Model file for the job. Use its own axes, mm. A direction names the side the tool comes from. Coordinates: 2 decimals unless noted, no trailing zeros. Order: outer loops, then holes, each group sorted by start corner. A loop starts at its lowest first (then second) coordinate and runs counter-clockwise, first axis right, second up. Notation, with made-up numbers: (-29.5, 4.5) -> (19.5, 4.5) arc R28 ccw to (19.5, 30.5) -> close; hole circle Ø8 at (2, 45). An arc over 180 degrees is marked (long way). Return JSON: item names as keys, results as strings. Group by question number.
1) Cut at C-C (y = -84.5). Write the cut outline in (x, z), and give its area (3 significant figures).
2) Pull direction Z, two halves, no side cores. Call faces 6 (the flat face through (9, -69, -6.5)), 7 (the flat face through (34, -77, 0)), 8 (the flat face through (-12.45, -87.22, -2.94)): +Z half, -Z half, draft (parallel to the pull), parting line (faces both ways), or undercut.
3) Cut at A-A (z = 0). Write the cut outline in (x, y).
4) Cut at B-B (x = -12). Write the cut outline in (y, z).
5) Cut at D-D (z = 5). Write the cut outline in (x, y), and give its area (3 significant figures).
6) Probe line 1 (Y direction, x = -6, z = 3); line 2 (X direction, y = -74.5, z = -2); line 3 (X direction, y = -88.5, z = 0). List the from-to ranges inside material, lowest first.
7) Flat gauge pins, fed straight in: pin 1 (4 mm diameter, centred on y = -81, z = 2.5, fed in from +X); pin 2 (3.5 mm diameter, centred on y = -86.5, z = -0.5, fed in from -X); pin 3 (4.5 mm diameter, centred on x = 34.5, z = 1.5, fed in from -Y); pin 4 (1 mm diameter, centred on x = 5, z = 4, fed in from -Y). Where does each tip first touch, or does it go through?
8) Which spindle directions (+Z, -Z, +X, -X, +Y, -Y) get a long thin tool onto all of the face, cutting with end or side? Do faces 1 (the flat face through (16, -62, 0)), 2 (the flat face through (-6.5, -87, 0)), 3 (the flat face through (-1, -82, 0)), 4 (the flat face through (-15, -50.15, 0)), 5 (the flat face through (34, -59, 0)). Say none if no direction does.
from build123d import *

# Parameters (mm, degrees)
BOSS_EXTRUDE1_START = -3
SKETCH1_W           = 13
SKETCH1_H           = 42.2
BOSS_EXTRUDE1_DEPTH = 2
BOSS_EXTRUDE2_START = -87.25
SKETCH2_R           = 6.5
BOSS_EXTRUDE2_DEPTH = 2.1
BOSS_EXTRUDE3_START = -87.25
SKETCH3_W           = 18.2
SKETCH3_H           = 13
BOSS_EXTRUDE3_DEPTH = 2.1
CUT_EXTRUDE1_START  = -87.25
SKETCH4_R           = 3.55
CUT_EXTRUDE1_DEPTH  = 2.1
CUT_EXTRUDE2_START  = -87.25
CUT_EXTRUDE2_DEPTH  = 2.1
BOSS_EXTRUDE4_START = -48.65
SKETCH6_R           = 6.5
BOSS_EXTRUDE4_DEPTH = 1.5
BOSS_EXTRUDE5_START = -48.65
SKETCH7_W           = 18.2
SKETCH7_H           = 13
BOSS_EXTRUDE5_DEPTH = 1.5
CUT_EXTRUDE3_START  = -48.65
SKETCH8_R           = 2.95
CUT_EXTRUDE3_DEPTH  = 1.5
BOSS_EXTRUDE6_START = 17
SKETCH9_W           = 13
SKETCH9_H           = 12
BOSS_EXTRUDE6_DEPTH = 19
BOSS_EXTRUDE7_START = 34
SKETCH10_W          = 13
SKETCH10_H          = 18
BOSS_EXTRUDE7_DEPTH = 2


with BuildPart() as part:
    # Sketch1 → Boss-Extrude1 (new, symmetric)
    with BuildSketch(Plane(origin=(0, 0, 0), x_dir=(0, 0, -1), z_dir=(1, 0, 0)).offset(BOSS_EXTRUDE1_START)):
        with Locations((0, -68.25)):
            Rectangle(SKETCH1_W, SKETCH1_H)
    extrude(amount=BOSS_EXTRUDE1_DEPTH, both=True)



with BuildPart() as body_2:
    # Sketch2 → Boss-Extrude2 (new, symmetric)
    with BuildSketch(Plane(origin=(0, 0, 0), x_dir=(1, 0, 0), z_dir=(0, 1, 0)).offset(BOSS_EXTRUDE2_START)):
        with Locations(Location((-19.2, 0, 0), (0, 0, 270))):
            Circle(SKETCH2_R)
    extrude(amount=BOSS_EXTRUDE2_DEPTH, both=True)


with BuildPart() as part_1:
    add(part.part)

    add(body_2.part)  # Boss-Extrude3 merges body 2
    # Sketch3 → Boss-Extrude3 (add, symmetric)
    with BuildSketch(Plane(origin=(0, 0, 0), x_dir=(1, 0, 0), z_dir=(0, 1, 0)).offset(BOSS_EXTRUDE3_START)):
        with Locations((-10.1, 0)):
            Rectangle(SKETCH3_W, SKETCH3_H)
    extrude(amount=BOSS_EXTRUDE3_DEPTH, both=True)

    # Sketch4 → Cut-Extrude1 (cut, symmetric)
    with BuildSketch(Plane(origin=(0, 0, 0), x_dir=(1, 0, 0), z_dir=(0, 1, 0)).offset(CUT_EXTRUDE1_START)):
        with Locations(Location((-19.2, 0, 0), (0, 0, 270))):
            Circle(SKETCH4_R)
    extrude(amount=CUT_EXTRUDE1_DEPTH, both=True, mode=Mode.SUBTRACT)

    # Sketch5 → Cut-Extrude2 (cut, symmetric)
    with BuildSketch(Plane(origin=(0, 0, 0), x_dir=(1, 0, 0), z_dir=(0, 1, 0)).offset(CUT_EXTRUDE2_START)):
        Polygon((-19.2, -3.55), (-6.5, -2.403281405), (-6.5, 2.403281405), (-19.2, 3.55), align=None)
    extrude(amount=CUT_EXTRUDE2_DEPTH, both=True, mode=Mode.SUBTRACT)



with BuildPart() as body_2_2:
    # Sketch6 → Boss-Extrude4 (new, symmetric)
    with BuildSketch(Plane(origin=(0, 0, 0), x_dir=(1, 0, 0), z_dir=(0, 1, 0)).offset(BOSS_EXTRUDE4_START)):
        with Locations(Location((-19.2, 0, 0), (0, 0, 270))):
            Circle(SKETCH6_R)
    extrude(amount=BOSS_EXTRUDE4_DEPTH, both=True)


with BuildPart() as part_2:
    add(part_1.part)

    add(body_2_2.part)  # Boss-Extrude5 merges body 2 2
    # Sketch7 → Boss-Extrude5 (add, symmetric)
    with BuildSketch(Plane(origin=(0, 0, 0), x_dir=(1, 0, 0), z_dir=(0, 1, 0)).offset(BOSS_EXTRUDE5_START)):
        with Locations((-10.1, 0)):
            Rectangle(SKETCH7_W, SKETCH7_H)
    extrude(amount=BOSS_EXTRUDE5_DEPTH, both=True)

    # Sketch8 → Cut-Extrude3 (cut, symmetric)
    with BuildSketch(Plane(origin=(0, 0, 0), x_dir=(1, 0, 0), z_dir=(0, 1, 0)).offset(CUT_EXTRUDE3_START)):
        with Locations(Location((-19.2, 0, 0), (0, 0, 270))):
            Circle(SKETCH8_R)
    extrude(amount=CUT_EXTRUDE3_DEPTH, both=True, mode=Mode.SUBTRACT)

    # Sketch9 → Boss-Extrude6 (add, symmetric)
    with BuildSketch(Plane(origin=(0, 0, 0), x_dir=(0, 0, -1), z_dir=(1, 0, 0)).offset(BOSS_EXTRUDE6_START)):
        with Locations((0, -68)):
            Rectangle(SKETCH9_W, SKETCH9_H)
    extrude(amount=BOSS_EXTRUDE6_DEPTH, both=True)

    # Sketch10 → Boss-Extrude7 (add, symmetric)
    with BuildSketch(Plane(origin=(0, 0, 0), x_dir=(0, 0, -1), z_dir=(1, 0, 0)).offset(BOSS_EXTRUDE7_START)):
        with Locations((0, -68)):
            Rectangle(SKETCH10_W, SKETCH10_H)
    extrude(amount=BOSS_EXTRUDE7_DEPTH, both=True)


solid = part_2.part
Answers below:
{
 "1": {"outline": "(-5, -6.5) -> (-1, -6.5) -> (-1, 6.5) -> (-5, 6.5) -> close", "area": "52.0 mm^2"},
 "2": {"face 6": "-Z half", "face 7": "draft", "face 8": "undercut"},
 "3": {"outline": "(-25.7, -89.35) -> (-22.75, -89.35) -> (-22.75, -85.15) -> (-25.7, -85.15) -> close; (-25.7, -50.15) -> (-22.15, -50.15) -> (-22.15, -47.15) -> (-25.7, -47.15) -> close; (-16.25, -50.15) -> (-5, -50.15) -> (-5, -85.15) -> (-6.5, -85.15) -> (-6.5, -89.35) -> (-1, -89.35) -> (-1, -74) -> (32, -74) -> (32, -77) -> (36, -77) -> (36, -59) -> (32, -59) -> (32, -62) -> (-1, -62) -> (-1, -47.15) -> (-16.25, -47.15) -> close"},
 "4": {"outline": "(-89.35, -6.5) -> (-85.15, -6.5) -> (-85.15, -2.9) -> (-89.35, -2.9) -> close; (-89.35, 2.9) -> (-85.15, 2.9) -> (-85.15, 6.5) -> (-89.35, 6.5) -> close; (-50.15, -6.5) -> (-47.15, -6.5) -> (-47.15, 6.5) -> (-50.15, 6.5) -> close"},
 "5": {"outline": "(-23.35, -89.35) -> (-1, -89.35) -> (-1, -74) -> (32, -74) -> (32, -77) -> (36, -77) -> (36, -59) -> (32, -59) -> (32, -62) -> (-1, -62) -> (-1, -47.15) -> (-23.35, -47.15) -> (-23.35, -50.15) -> (-5, -50.15) -> (-5, -85.15) -> (-23.35, -85.15) -> close", "area": "769 mm^2"},
 "6": {"line 1": "y = -89.35 to -85.15, -50.15 to -47.15", "line 2": "x = -5 to -1, 32 to 36", "line 3": "x = -25.7 to -22.75, -6.5 to -1"},
 "7": {"pin 1": "stops at x = -1", "pin 2": "stops at x = -25.7", "pin 3": "stops at y = -77", "pin 4": "stops at y = -74"},
 "8": {"face 1": "+Z, -Z, +Y", "face 2": "-Y", "face 3": "+Z, -Z, -Y", "face 4": "+Z, -Z, -X", "face 5": "+Z, -Z, +X, +Y"}
}
